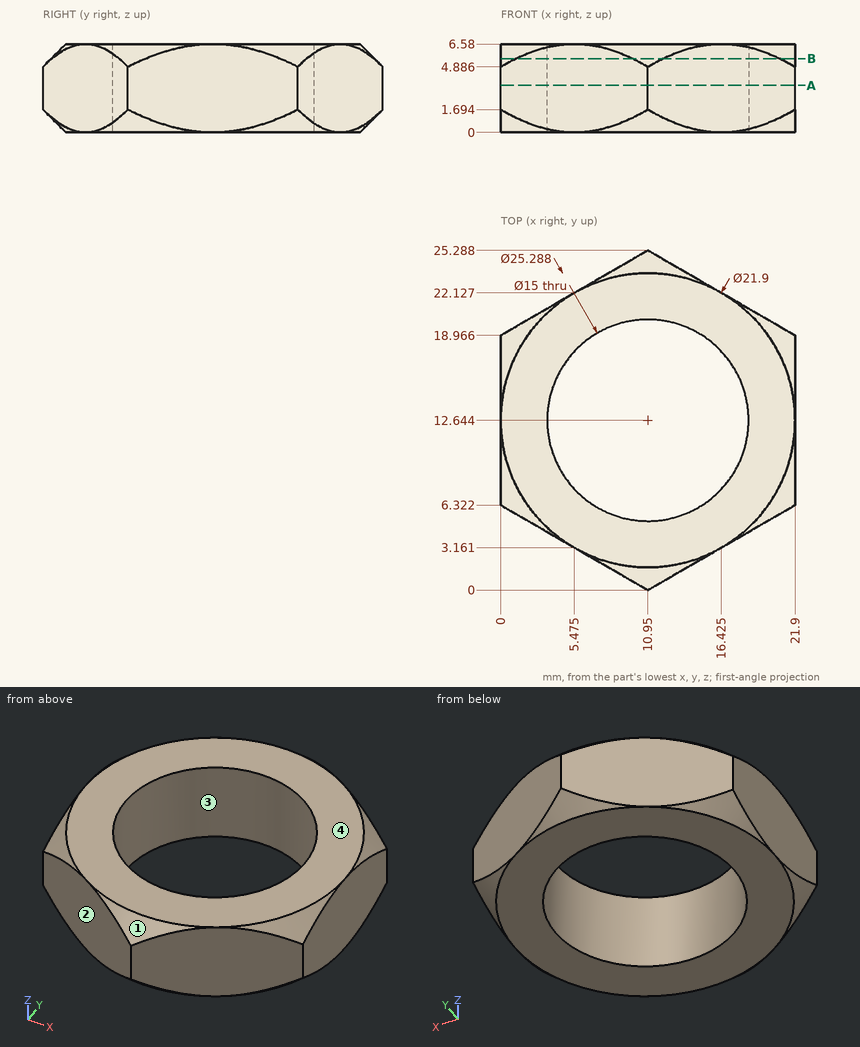
For this review, use the dimensioned drawing (mm, ordinates from the lowest corner) and the shaded views. Round coordinates to 2 decimals unless told otherwise and drop trailing zeros. Order: outer loops, then holes, each group sorted by start corner. A loop starts at its lowest first (then second) coordinate and runs counter-clockwise, first axis right, second up. Notation, with made-up numbers: (87, 29.5) -> (94, 29.5) arc R30 cw to (94, 62.5) -> close; hole circle Ø2 at (5, 23). An arc over 180 degrees is marked (long way). Write item = value, one per line. Start each with the question number.
Item 1: Consider section A-A on z = 3.5. Write out the cut boundary in (x, y).
Item 2: Mouldability with a two-part tool opening along X and no side actions: class the marked faces 1, 2, 3 and 4 as released by +X, released by -X, zero draft, split by the parting line, or undercut.
Item 3: For line 1 along X through (y, z) = (12.5, 5.75); line 2 along Y through (x, z) = (10.95, 1.5); line 3 along Y through (x, z) = (14, 3), list the stretches that pass through material, from the lowest coordinate up.
Item 4: Clearance check with flat-ended pins moving along their axes: pin 1 Ø9 at (x, y) = (10.95, 12.64) entering from +Z; pin 2 Ø3 at (x, z) = (3.5, 1.5) entering from -Y. State where each tip first meets the part, or that it passes through.
Item 5: Consider section B-B on z = 5.5. Write out the cut boundary in (x, y), plus the area to 4 significant figures.
Conclusion:
q1.outline = (0, 6.32) -> (10.95, 0) -> (21.9, 6.32) -> (21.9, 18.97) -> (10.95, 25.29) -> (0, 18.97) -> close; hole circle Ø15 at (10.95, 12.64)
q2.face_1 = split by the parting line
q2.face_2 = released by -X
q2.face_3 = undercut
q2.face_4 = zero draft
q3.line_1 = 0 to 3.45, 18.45 to 21.9
q3.line_2 = 0.19 to 5.14, 20.14 to 25.09
q3.line_3 = 1.76 to 5.79, 19.5 to 23.53
q4.pin_1 = through
q4.pin_2 = 3.44
q5.outline = (0, 7.66) arc R12.03 ccw to (1.16, 5.65) -> (9.79, 0.67) arc R12.03 ccw to (12.11, 0.67) -> (20.74, 5.65) arc R12.03 ccw to (21.9, 7.66) -> (21.9, 17.63) arc R12.03 ccw to (20.74, 19.64) -> (12.11, 24.62) arc R12.03 ccw to (9.79, 24.62) -> (1.16, 19.64) arc R12.03 ccw to (0, 17.63) -> close; hole circle Ø15 at (10.95, 12.64)
q5.area = 234.5 mm2
